from build123d import *

# Parameters (mm, degrees)
SKETCH1_W           = 20
SKETCH1_H           = 33
SKETCH1_W_2         = 17
SKETCH1_H_2         = 30
BOSS_EXTRUDE1_DEPTH = 35
SKETCH2_W           = 20
SKETCH2_H           = 33
BOSS_EXTRUDE2_DEPTH = 1
SKETCH3_W           = 1.5
SKETCH3_H           = 2
BOSS_EXTRUDE3_DEPTH = 35


with BuildPart() as part:
    # Sketch1 → Boss-Extrude1 (new body)
    with BuildSketch(Plane(origin=(0, 0, 0), x_dir=(1, 0, 0), z_dir=(0, 1, 0))):
        Rectangle(SKETCH1_W, SKETCH1_H)
        Rectangle(SKETCH1_W_2, SKETCH1_H_2, mode=Mode.SUBTRACT)
    extrude(amount=BOSS_EXTRUDE1_DEPTH)

    # Sketch2 → Boss-Extrude2 (add)
    with BuildSketch(Plane(origin=(0, 35, 0), x_dir=(1, 0, 0), z_dir=(0, 1, 0))):
        Rectangle(SKETCH2_W, SKETCH2_H)
    extrude(amount=BOSS_EXTRUDE2_DEPTH)

    # Sketch3 → Boss-Extrude3 (add)
    with BuildSketch(Plane.XZ):
        with Locations((-2.75, -14)):
            Rectangle(SKETCH3_W, SKETCH3_H)
        with Locations((2.75, -14)):
            Rectangle(SKETCH3_W, SKETCH3_H)
        with Locations((2.75, 14)):
            Rectangle(SKETCH3_W, SKETCH3_H)
        with Locations((-2.75, 14)):
            Rectangle(SKETCH3_W, SKETCH3_H)
    extrude(amount=-BOSS_EXTRUDE3_DEPTH)


solid = part.part
Geometry: final body of the model. Coordinates: model frame, mm. A direction names the side the tool comes from. Give positions to 0.01 mm unless a question says otherwise; leave off trailing zeros. Write each loop counter-clockwise with the first axis right and the second up, starting at its lowest first coordinate (ties: lowest second). Pieces come first, ordered by that corner, then holes.
(1) Access query for faces 4 (the flat face through (0, 36, 0)), 5 (the flat face through (3, 17, 13)). Directions: +Z, -Z, +X, -X, +Y, -Y. A direction counts if a zero-diameter tool reaches every point of the face in a straight line with its end or side. Return the directions, or none.
(2) Ray query, line 1 (Z direction, x = 5.5, y = 9.5); line 2 (X direction, y = 3.5, z = -12); line 3 (Z direction, x = -3, y = 30.5). Return the intervals inside material, ascending.
(3) Cut plane A-A, the plane y = 22. Return loops of the section in (x, z), then the cut area to 3 significant figures.
(4) Cut plane B-B, the plane z = 3. Return loops of the section in (x, y), then the cut area to 3 significant figures.
(5) Mould query, pull axis X, two halves, no side actions, for faces 1 (the flat face through (0, 18, -16.5)), 2 (the flat face through (10, 18, 0)), 3 (the flat face through (-8.5, 17, 0)). Classes: released by +X, released by -X, zero draft, split by the parting line, or undercut.
(6) Cut plane C-C, the plane x = -6.5. Return loops of the section in (y, z).
(7) First-contact query: P1, Ø8.5, axis at x = 3, z = 0, coming from the -Y side. Flat tip, straight axial feed; report the tip coordinate or a pass-through.
(8) Cut plane D-D, the plane z = -14. Return loops of the section in (x, y).
Values follow:
1. face 4: +Z, -Z, +X, -X, +Y
1. face 5: -Y
2. line 1: z = -16.5 to -15, 15 to 16.5
2. line 2: x = -10 to -8.5, 8.5 to 10
2. line 3: z = -16.5 to -13, 13 to 16.5
3. outline: (-10, -16.5) - (10, -16.5) - (10, 16.5) - (-10, 16.5) - close; hole (-8.5, -15) - (-3.5, -15) - (-3.5, -13) - (-2, -13) - (-2, -15) - (2, -15) - (2, -13) - (3.5, -13) - (3.5, -15) - (8.5, -15) - (8.5, 15) - (3.5, 15) - (3.5, 13) - (2, 13) - (2, 15) - (-2, 15) - (-2, 13) - (-3.5, 13) - (-3.5, 15) - (-8.5, 15) - close
3. area: 162 mm2
4. outline: (-10, 0) - (-8.5, 0) - (-8.5, 35) - (8.5, 35) - (8.5, 0) - (10, 0) - (10, 36) - (-10, 36) - close
4. area: 125 mm2
5. face 1: zero draft
5. face 2: released by +X
5. face 3: undercut
6. outline: (0, -16.5) - (36, -16.5) - (36, 16.5) - (0, 16.5) - (0, 15) - (35, 15) - (35, -15) - (0, -15) - close
7. P1: stops at y = 35
8. outline: (-10, 0) - (-8.5, 0) - (-8.5, 35) - (-3.5, 35) - (-3.5, 0) - (-2, 0) - (-2, 35) - (2, 35) - (2, 0) - (3.5, 0) - (3.5, 35) - (8.5, 35) - (8.5, 0) - (10, 0) - (10, 36) - (-10, 36) - close
